The figure shows three views and two pictorial views of one solid part (mm, origin at its lowest corner). Answer the questions. Coordinates: 2 decimals unless noted, no trailing zeros. Order: outer loops, then holes, each group sorted by start corner. A loop starts at its lowest first (then second) coordinate and runs counter-clockwise, first axis right, second up.
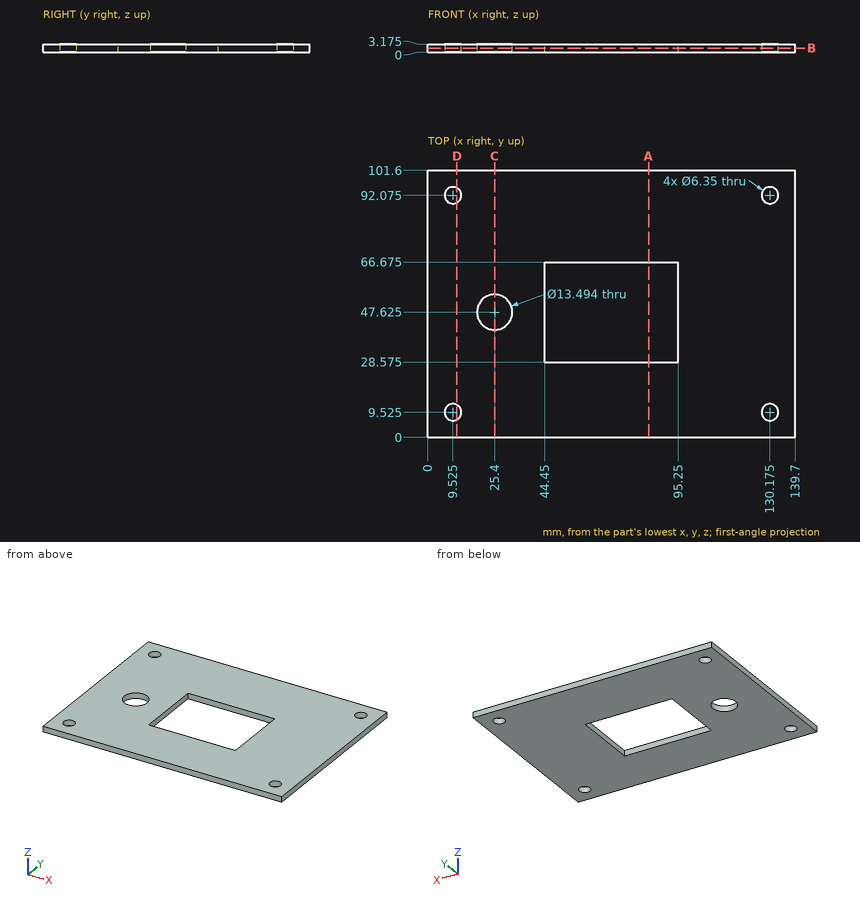
1) A cutting plane is placed at D-D, the plane x = 11. Write down the section's boundary in (y, z) (1 decimal), plus the area to 3 significant figures.
2) Each of these flat-tipped pins is pushed along its axis until it touches: P1, Ø15.5, axis at x = 25.4, y = 47.625, coming from the +Z side (3 decimals); P2, Ø2, axis at x = 68, y = 30, coming from the -Z side. Where does it stop, or does it pass through?
3) A cutting plane is placed at C-C, the plane x = 25.4. Write down the section's boundary in (y, z) (1 decimal), plus the area to 3 significant figures.
4) A cutting plane is placed at A-A, the plane x = 84. Write down the section's boundary in (y, z) (1 decimal).
5) Straight lines are drawn through the part: probe 1 along Y at (x, z) = (86.5, 1.3) (1 decimal); probe 2 along X at (y, z) = (47, 2.75); probe 3 along X at (y, z) = (34, 1.8). For each, find the intervals that lie inside material, in ascending order.
6) A cutting plane is placed at B-B, the plane z = 1.65. Count the separate pieces of the cut face and the enclosed holes in it, plus the area to 3 significant figures.
Working result:
1. outline: (0, 0) - (6.7, 0) - (6.7, 3.2) - (0, 3.2) - close; (12.3, 0) - (89.3, 0) - (89.3, 3.2) - (12.3, 3.2) - close; (94.9, 0) - (101.6, 0) - (101.6, 3.2) - (94.9, 3.2) - close
1. area: 287 mm2
2. P1: stops at z = 3.175
2. P2: passes through
3. outline: (0, 0) - (40.9, 0) - (40.9, 3.2) - (0, 3.2) - close; (54.4, 0) - (101.6, 0) - (101.6, 3.2) - (54.4, 3.2) - close
3. area: 280 mm2
4. outline: (0, 0) - (28.6, 0) - (28.6, 3.2) - (0, 3.2) - close; (66.7, 0) - (101.6, 0) - (101.6, 3.2) - (66.7, 3.2) - close
5. probe 1: y = 0 to 28.6, 66.7 to 101.6
5. probe 2: x = 0 to 18.68, 32.12 to 44.45, 95.25 to 139.7
5. probe 3: x = 0 to 44.45, 95.25 to 139.7
6. separate pieces: 1
6. enclosed holes: 6
6. area: 12,000 mm2
